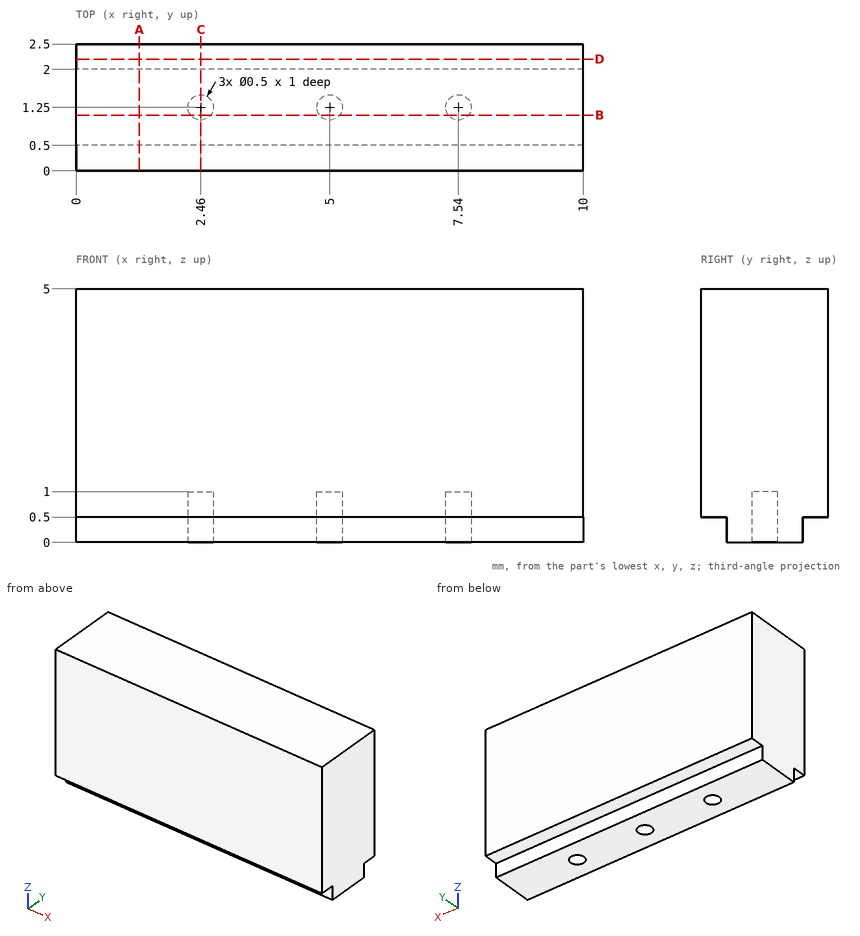
Could you check a few things on this drawing? It's one solid part, dimensions in mm from its lowest x, y, z. Coordinates: 2 decimals unless noted, no trailing zeros. Write each loop counter-clockwise with the first axis right and the second up, starting at its lowest first coordinate (ties: lowest second). Pieces come first, ordered by that corner, then holes. Notation, with made-up numbers: M -2.5,51 L 21.5,51 A23 cw 21.5,82 Z; hole C -34,57 d2. An arc over 180 degrees is marked long. One line per question, with ' | ' between items.
1) Imagine slicing it at B-B, the plane y = 1.1. Write out the boundary of the cut face in (x, z).
Checks:
outline: M 0,0 L 2.26,0 L 2.26,1 L 2.66,1 L 2.66,0 L 4.8,0 L 4.8,1 L 5.2,1 L 5.2,0 L 7.34,0 L 7.34,1 L 7.74,1 L 7.74,0 L 10,0 L 10,5 L 0,5 Z
2) I need wall thicknesses on probe 1 along Y at (x, z) = (7.54, 0.75); probe 2 along Z at (x, y) = (4, 0.35); probe 3 along Y at (x, z) = (2.46, 0.3). Which ranges of each line are inside material? Lowest first, please. Write a range as [from, to].
Checks:
probe 1: [0, 1], [1.5, 2.5] | probe 2: [0.5, 5] | probe 3: [0.5, 1], [1.5, 2]
3) Imagine slicing it at C-C, the plane x = 2.46. Write out the boundary of the cut face in (y, z), and give its area (3 significant figures).
Checks:
outline: M 0,0.5 L 0.5,0.5 L 0.5,0 L 1,0 L 1,1 L 1.5,1 L 1.5,0 L 2,0 L 2,0.5 L 2.5,0.5 L 2.5,5 L 0,5 Z | area: 11.5 mm²
4) Imagine slicing it at A-A, the plane x = 1.25. Write out the boundary of the cut face in (y, z), and give its area (3 significant figures).
Checks:
outline: M 0,0.5 L 0.5,0.5 L 0.5,0 L 2,0 L 2,0.5 L 2.5,0.5 L 2.5,5 L 0,5 Z | area: 12.0 mm²
5) For pin 1 Ø1 at (x, z) = (5.5, 2.5) entering from -Y; pin 2 Ø0.6 at (x, z) = (3.5, 0) entering from -Y, each with a flat end and sliding along its axis, tell me the tip position at first contact or that it passes through.
Checks:
pin 1: y = 0 | pin 2: y = 0.5
6) Imagine slicing it at D-D, the plane y = 2.2. Write out the boundary of the cut face in (x, z).
Checks:
outline: M 0,0.5 L 10,0.5 L 10,5 L 0,5 Z
